Here's how the part is built. I have some questions about the finished solid (model axes, mm). Face numbers are marked on the shaded views. A direction names the side the tool comes from. Round coordinates to 2 decimals unless told otherwise and drop trailing zeros. Write each loop counter-clockwise with the first axis right and the second up, starting at its lowest first coordinate (ties: lowest second). Pieces come first, ordered by that corner, then holes. Notation, with made-up numbers: M 16,30.25 L 43,30.25 A19 ccw 43,47.25 Z; hole C -14,-16.5 d6. An arc over 180 degrees is marked long. Use one line per item in the form item = value. Start each with the question number.
Q1. I want a section at C-C on y = -43.9. List the corners of the cut face in (x, z) for me, and give its area (3 significant figures).
Q2. I'm going to push flat-ended pins straight in: pin 1 Ø7 at (x, y) = (44, -43) entering from +Z; pin 2 Ø10 at (x, z) = (33, 69.5) entering from -Y; pin 3 Ø12 at (x, y) = (-16.5, 40.5) entering from +Z; pin 4 Ø8 at (x, z) = (37.5, 50) entering from +Y. Where does each tip first touch, or does it pass through?
Q3. For the marked faces 1 and 2, which set-ups out of +Z, -Z, +X, -X, +Y, -Y let a thin tool reach every point of the face, with its end or its side?
Q4. I want a section at B-B on x = -36.5. List the corners of the cut face in (y, z) for me.
Q5. I want a section at A-A on y = 0. List the corners of the cut face in (x, z) for me, and give its area (3 significant figures).
Q6. I need wall thicknesses on line 1 along X through (y, z) = (-43.9, 44.15); line 2 along Y through (x, z) = (-51.9, 40.1). Which ranges of each line are inside material? Lowest first, please. Write a range as from..to.
```python
from build123d import *

# Parameters (mm, degrees)
PAD013_DEPTH          = 2
SKETCH027_R           = 2
POCKET011_DEPTH       = 2
CHAMFER004_SIZE       = 1
SKETCH028_R           = 30
POCKET012_DEPTH       = 5
SKETCH029_R           = 32.5
SKETCH029_R_2         = 30
PAD014_DEPTH          = 96
SKETCH030_W           = 14
SKETCH030_H           = 6
POCKET013_DEPTH       = 5
POLARPATTERN007_COUNT = 6
SKETCH031_W           = 14
SKETCH031_H           = 6
POCKET014_DEPTH       = 5
POLARPATTERN008_COUNT = 6
SKETCH032_R           = 5
SKETCH032_R_2         = 3.1
PAD015_DEPTH          = 4
POLARPATTERN009_COUNT = 4


with BuildPart() as part:
    # Sketch026 → Pad013 (new body)
    with BuildSketch(Plane.XY):
        with BuildLine():
            Line((-51.9, -57.9), (51.9, -57.9))
            ThreePointArc((51.9, -57.9), (56.1426406871, -56.1426406871), (57.9, -51.9))
            Line((57.9, -51.9), (57.9, 51.9))
            ThreePointArc((57.9, 51.9), (56.1426406871, 56.1426406871), (51.9, 57.9))
            Line((51.9, 57.9), (-51.9, 57.9))
            ThreePointArc((-51.9, 57.9), (-56.1426406871, 56.1426406871), (-57.9, 51.9))
            Line((-57.9, 51.9), (-57.9, -51.9))
            ThreePointArc((-57.9, -51.9), (-56.1426406871, -56.1426406871), (-51.9, -57.9))
        make_face()
    extrude(amount=PAD013_DEPTH)

    # Sketch027 (on Face10 of Pad013) → Pocket011 (cut)
    with BuildSketch(Plane.XY.offset(2)):
        with Locations((-51.900002, 51.900002)):
            Circle(SKETCH027_R)
        with Locations((51.9, 51.9)):
            Circle(SKETCH027_R)
        with Locations((51.9, -51.9)):
            Circle(SKETCH027_R)
        with Locations((-51.9, -51.9)):
            Circle(SKETCH027_R)
    extrude(amount=-POCKET011_DEPTH, mode=Mode.SUBTRACT)

    # Chamfer004
    chamfer004_edges = [part.edges().sort_by_distance(p)[0] for p in [
        (-53.9, -51.9, 2),
        (-53.900002, 51.900002, 2),
        (49.9, 51.9, 2),
        (49.9, -51.9, 2),
    ]]
    chamfer(chamfer004_edges, length=CHAMFER004_SIZE)

    # Sketch028 (on Face1 of Chamfer004) → Pocket012 (cut)
    with BuildSketch(Plane.XY.offset(2)):
        Circle(SKETCH028_R)
    extrude(amount=-POCKET012_DEPTH, mode=Mode.SUBTRACT)

    # Sketch029 (on Face1 of Pocket012) → Pad014 (join)
    with BuildSketch(Plane.XY.offset(2)):
        Circle(SKETCH029_R)
        Circle(SKETCH029_R_2, mode=Mode.SUBTRACT)
    extrude(amount=PAD014_DEPTH)

    # Sketch030 (on Face1 of Pad014) → Pocket013 (cut)
    with BuildSketch(Plane.XY.offset(2)):
        with Locations((0, 39)):
            Rectangle(SKETCH030_W, SKETCH030_H)
    pocket013 = extrude(amount=-POCKET013_DEPTH, mode=Mode.SUBTRACT)

    # PolarPattern007: Pocket013 ×6 about axis
    polarpattern007_axis = Axis((0, 0, 2), (0, 0, 1))
    for i in range(1, POLARPATTERN007_COUNT):
        add(pocket013.rotate(polarpattern007_axis, i * 360 / POLARPATTERN007_COUNT), mode=Mode.SUBTRACT)

    # Sketch031 (on Face42 of PolarPattern007) → Pocket014 (cut)
    with BuildSketch(Plane.XY.offset(98)):
        with Locations((0, 31)):
            Rectangle(SKETCH031_W, SKETCH031_H)
    pocket014 = extrude(amount=-POCKET014_DEPTH, mode=Mode.SUBTRACT)

    # PolarPattern008: Pocket014 ×6 about axis
    polarpattern008_axis = Axis((0, 0, 98), (0, 0, 1))
    for i in range(1, POLARPATTERN008_COUNT):
        add(pocket014.rotate(polarpattern008_axis, i * 360 / POLARPATTERN008_COUNT), mode=Mode.SUBTRACT)

    # Sketch032 (on Face1 of PolarPattern008) → Pad015 (join)
    with BuildSketch(Plane.XY.offset(2)):
        with Locations((-43.9, 43.9)):
            Circle(SKETCH032_R)
        with Locations((-43.9, 43.9)):
            Circle(SKETCH032_R_2, mode=Mode.SUBTRACT)
    pad015 = extrude(amount=PAD015_DEPTH)

    # PolarPattern009: Pad015 ×4 about axis
    polarpattern009_axis = Axis((0, 0, 2), (0, 0, 1))
    for i in range(1, POLARPATTERN009_COUNT):
        add(pad015.rotate(polarpattern009_axis, i * 360 / POLARPATTERN009_COUNT))


with BuildPart() as part_1:
    # Body003 placement: moved
    add(part.part.moved(Location((0, 0, 39.5))))


solid = part_1.part
```
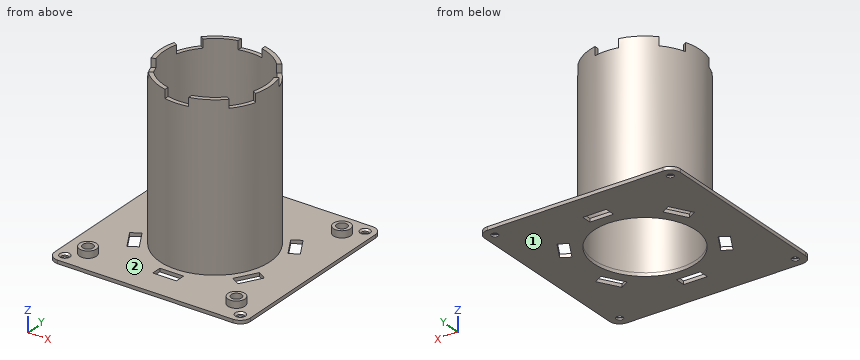
Reported:
q1.outline = M -57.9,39.5 L 57.9,39.5 L 57.9,41.5 L 48.9,41.5 L 48.9,45.5 L 47,45.5 L 47,41.5 L 40.8,41.5 L 40.8,45.5 L 38.9,45.5 L 38.9,41.5 L -38.9,41.5 L -38.9,45.5 L -40.8,45.5 L -40.8,41.5 L -47,41.5 L -47,45.5 L -48.9,45.5 L -48.9,41.5 L -57.9,41.5 Z
q1.area = 262 mm^2
q2.pin_1 = 45.5
q2.pin_2 = -16.5
q2.pin_3 = 41.5
q2.pin_4 = through
q3.face_1 = -Z, +X, -X, +Y, -Y
q3.face_2 = +Z
q4.outline = M -57.9,39.5 L -20.78,39.5 L -20.78,41.5 L -57.9,41.5 Z; M -12.99,39.5 L 12.99,39.5 L 12.99,41.5 L -12.99,41.5 Z; M 20.78,39.5 L 57.9,39.5 L 57.9,41.5 L 20.78,41.5 Z
q5.outline = M -57.9,39.5 L -30,39.5 L -30,137.5 L -32.5,137.5 L -32.5,41.5 L -57.9,41.5 Z; M 30,39.5 L 57.9,39.5 L 57.9,41.5 L 32.5,41.5 L 32.5,137.5 L 30,137.5 Z
q5.area = 592 mm^2
q6.line_1 = -48.9..-47, -40.8..-38.9, 38.9..40.8, 47..48.9
q6.line_2 = -57.9..-53.9, -49.9..49.9, 53.9..57.9
